Source: CAD feature listing. Evaluate the final solid. Frame: model axes, mm. A direction names the side the tool comes from. Give positions to 0.01 mm unless a question says otherwise; leave off trailing zeros. Write each loop counter-clockwise with the first axis right and the second up, starting at its lowest first coordinate (ties: lowest second). Pieces come first, ordered by that corner, then holes. Notation, with made-up numbers: (89.5, -15) -> (108.5, -15) arc R17 ccw to (108.5, -9) -> close; hole circle Ø8 at (69.25, -16). An arc over 180 degrees is marked (long way). Use one line per item in the form item = value. Start each with the question number.
(1) Cut plane D-D, the plane z = -20.5. Output: boundary loops of the cut face in (x, y).
(2) Cut plane A-A, the plane z = -6.25. Output: boundary loops of the cut face in (x, y).
(3) Set-up query: faces 4 (the face through (35, 0, -12)), 5 (the face through (-35.645, 0.154, 0.572)). Return all of +Z, -Z, +X, -X, +Y, -Y with unobstructed straight access to the full face (end or side cutting, diameter ignored); none if empty.
(4) Material intervals for line 1 along X through (y, z) = (5.75, -23); line 2 along Y through (x, z) = (-25, 0.6); line 3 along Y through (x, z) = (36.55, -18), sorted ascending. Write a range as from..to.
(5) Cut plane B-B, the plane x = 25. Output: boundary loops of the cut face in (y, z).
(6) Draft query along X for faces 1 (the face through (35.645, -0.154, 0.572)), 2 (the face through (-37, 3, -13)), 3 (the face through (-35, 0, -12)). Return one class per face: pulls with the +X half, pulls with the -X half, needs draft (parallel to the pull), parting line crosses it, or undercut.
(7) Cut plane C-C, the plane y = 0. Output: boundary loops of the cut face in (x, z), and give its area (3 significant figures).
(8) First-contact query: P1, Ø12, axis at x = 17.5, y = 3.5, coming from the -Z side. Flat tip, straight axial feed; report the tip coordinate or a pass-through.
Autodesk Inventor part; units mm, degrees
ref_plane "YZ Plane" through (0, 0, 0) normal (1, 0, 0) x (0, 1, 0)
ref_plane "XZ Plane" through (0, 0, 0) normal (0, 1, 0) x (-1, 0, 0)
ref_plane "XY Plane" through (0, 0, 0) normal (0, 0, 1) x (1, 0, 0)
sketch "Sketch1" plane through (0, 0, 0) normal (0, 0, 1) x (1, 0, 0)
  line L0 (-35, -11) -> (35, -11)
  line L1 (35, -11) -> (35, 11)
  line L2 (35, 11) -> (-35, 11)
  line L3 (-35, 11) -> (-35, -11)
  line L4 (-35, -11) -> (35, 11) construction
  line L5 (35, -11) -> (-35, 11) construction
  circle A0 centre (-25, 0) radius 2.75
  circle A1 centre (25, 0) radius 2.75
  line L6 (0, 11) -> (0, -18.7198) construction
  point P0 (0, 0)
  dimension "d154" = 70
  dimension "d155" = 22
  dimension "d197" = 50
  dimension "d198" = 5.5
extrude "Plate5" add sketch "Sketch1" along normal blind 2
sketch "Sketch10" plane through (-37, 11, 2) normal (1, 0, 0) x (0, 1, 0)
  line L0 (-22, 0) -> (0, 0)
  line L1 (0, 0) -> (0, -30)
  line L2 (0, -30) -> (-22, -30)
  line L3 (-22, -30) -> (-22, 0)
edge flange "Flange4" height 30 angle 90 thickness 2 bend radius 2.75 thickness toward (1, 0, 0) relief round relief width 2 relief depth 1 corner gap 2.75 corner form 0 edges at (-35, 0, 0) (35, 0, 0) wall of the first edge with corners at (-37, -11, 2) (-37, 11, 2) (-37, 11, -28) (-37, -11, -28)
bend "Bend4"
corner "Corner4"
sketch "Sketch11" plane through (-35, -11, -28) normal (1, 0, 0) x (0, 0, -1)
  line L0 (-25.25, 22) -> (-25.25, 0) construction
  line L1 (-25.25, 0) -> (0, 0) construction
  line L2 (0, 0) -> (0, 22) construction
  line L3 (-25.25, 22) -> (0, 22) construction
  circle A0 centre (-10, 11) radius 5.5
  point P0 (-28, 11)
  point P1 (0, 11)
  dimension "d192" = 11
  dimension "d193" = 10
extrude "Cut3" cut sketch "Sketch11" against normal blind 2
mirror "Mirror1" about plane through (0, 0, 0) normal (1, 0, 0) of "Cut3"
fillet "Corner Round3" radius 6 4 edges at (-36, 11, -28) (-36, -11, -28) (36, -11, -28) (36, 11, -28)
properties part number "TKS 3525 FDS diam support" material "Stainless Steel"
Geometry says:
q1.outline = (-37, -11) -> (-35, -11) -> (-35, -4.9) -> (-37, -4.9) -> close; (-37, 4.9) -> (-35, 4.9) -> (-35, 11) -> (-37, 11) -> close; (35, -11) -> (37, -11) -> (37, -4.9) -> (35, -4.9) -> close; (35, 4.9) -> (37, 4.9) -> (37, 11) -> (35, 11) -> close
q2.outline = (-37, -11) -> (-35, -11) -> (-35, 11) -> (-37, 11) -> close; (35, -11) -> (37, -11) -> (37, 11) -> (35, 11) -> close
q3.face_4 = -Z, +Y, -Y
q3.face_5 = +Z, -X, +Y, -Y
q4.line_1 = -37..-35, 35..37
q4.line_2 = -11..-2.75, 2.75..11
q4.line_3 = -11..-5.5, 5.5..11
q5.outline = (-11, 0) -> (-2.75, 0) -> (-2.75, 2) -> (-11, 2) -> close; (2.75, 0) -> (11, 0) -> (11, 2) -> (2.75, 2) -> close
q6.face_1 = pulls with the +X half
q6.face_2 = pulls with the -X half
q6.face_3 = undercut
q7.outline = (-37, -28) -> (-35, -28) -> (-35, -23.5) -> (-37, -23.5) -> close; (-37, -12.5) -> (-35, -12.5) -> (-35, -2.75) arc R2.75 cw to (-32.25, 0) -> (-27.75, 0) -> (-27.75, 2) -> (-32.25, 2) arc R4.75 ccw to (-37, -2.75) -> close; (-22.25, 0) -> (22.25, 0) -> (22.25, 2) -> (-22.25, 2) -> close; (27.75, 0) -> (32.25, 0) arc R2.75 cw to (35, -2.75) -> (35, -12.5) -> (37, -12.5) -> (37, -2.75) arc R4.75 ccw to (32.25, 2) -> (27.75, 2) -> close; (35, -28) -> (37, -28) -> (37, -23.5) -> (35, -23.5) -> close
q7.area = 188 mm^2
q8.P1 = 0
